Design review of the part built by this model. Coordinates are the model's own, in mm. Face numbers are marked on the shaded views. A direction names the side the tool comes from. Coordinates: 2 decimals unless noted, no trailing zeros. Loops run counter-clockwise (first coordinate to the right, second up) from the corner with the lowest first, then second, coordinate; pieces in that order, holes last. Notation, with made-up numbers: M 84,66 L 121,66 A9 cw 121,80 Z; hole C 14.25,51.5 d8. An arc over 180 degrees is marked long. Write item = value, one per line. Start each with the question number.
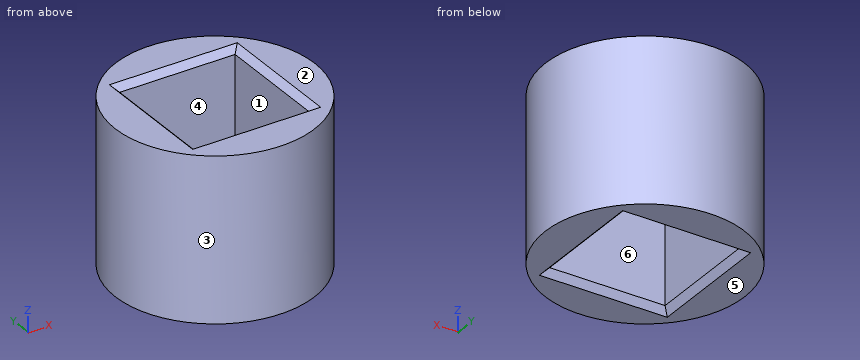
from build123d import *

# Parameters (mm, degrees)
SKETCH1_R           = 3.175
SKETCH1_W           = 3.675
SKETCH1_H           = 3.675
BOSS_EXTRUDE1_DEPTH = 5.188
CHAMFER1_SIZE       = 0.2


with BuildPart() as part:
    # Sketch1 → Boss-Extrude1 (new body)
    with BuildSketch(Plane.XY):
        Circle(SKETCH1_R)
        Rectangle(SKETCH1_W, SKETCH1_H, mode=Mode.SUBTRACT)
    extrude(amount=BOSS_EXTRUDE1_DEPTH)

    # Chamfer1
    chamfer1_edges = [part.edges().sort_by_distance(p)[0] for p in [
        (0, -1.8375, 5.188),
        (1.8375, 0, 0),
        (0, 1.8375, 0),
        (-1.8375, 0, 0),
        (0, -1.8375, 0),
        (1.8375, 0, 5.188),
        (0, 1.8375, 5.188),
        (-1.8375, 0, 5.188),
    ]]
    chamfer(chamfer1_edges, length=CHAMFER1_SIZE)


solid = part.part
Q1. For the marked faces 5 and 6, list the 3-axis set-ups (+Z, -Z, +X, -X, +Y, -Y) from which the entire face can be reached by the end or side of a thin tool; tool diameter is ignored.
Q2. Add section D-D on x = -2.25. State the section outline as (y, z) points, plus the area to 3 significant figures.
Q3. To check wall thickness, follow line 1 (Y direction, x = 0, z = 4.05) (1 decimal); line 2 (Y direction, x = -1, z = 2.3); line 3 (X direction, y = 0.5, z = 4.5). State the ranges of each line that lie inside material, in increasing order. Write a range as from..to.
Q4. Mouldability with a two-part tool opening along X and no side actions: class the marked faces 1, 2, 3 and 4 as released by +X, released by -X, zero draft, split by the parting line, or undercut.
Q5. Clearance check with flat-ended pins moving along their axes: P1, Ø1.5, axis at x = -1.5, z = 2, coming from the +Y side; P2, Ø3, axis at x = -0.5, z = 2.5, coming from the +Y side (3 decimals); P3, Ø1, axis at y = -1, z = 2, coming from the -X side; P4, Ø1, axis at y = -2, z = 2.5, coming from the +X side. State where each tip first meets the part, or that it passes through.
Values follow:
q1.face_5 = -Z, +X, -X, +Y, -Y
q1.face_6 = +Z, -Z
q2.outline = M -2.24,0 L 2.24,0 L 2.24,5.19 L -2.24,5.19 Z
q2.area = 23.2 mm2
q3.line_1 = -3.2..-1.8, 1.8..3.2
q3.line_2 = -3.01..-1.84, 1.84..3.01
q3.line_3 = -3.14..-1.84, 1.84..3.14
q4.face_1 = undercut
q4.face_2 = zero draft
q4.face_3 = split by the parting line
q4.face_4 = undercut
q5.P1 = 3.09
q5.P2 = 3.175
q5.P3 = -3.14
q5.P4 = 2.8
